from build123d import *

# Parameters (mm, degrees)
SKETCH_1_R      = 1.5
EXTRUDE_1_DEPTH = 14
FILLET_1_R      = 0.5


with BuildPart() as part:
    # 草图1 → 凸台-拉伸1 (new body)
    with BuildSketch(Plane(origin=(0, 0, 0), x_dir=(1, 0, 0), z_dir=(0, 1, 0))):
        Polygon((2.3, -1.327905619), (2.3, 1.327905619), (0, 2.655811238), (-2.3, 1.327905619), (-2.3, -1.327905619), (0, -2.655811238), align=None)
        Circle(SKETCH_1_R, mode=Mode.SUBTRACT)
    extrude(amount=EXTRUDE_1_DEPTH)

    # 圆角1
    fillet_1_edges = [part.edges().sort_by_distance(p)[0] for p in [
        (1.15, 14, -1.991858429),
        (-1.15, 14, -1.991858429),
        (-2.3, 14, 0),
        (-1.15, 14, 1.991858429),
        (1.15, 14, 1.991858429),
        (-1.15, 0, 1.991858429),
        (-2.3, 0, 0),
        (-1.15, 0, -1.991858429),
        (1.15, 0, -1.991858429),
        (2.3, 0, 0),
        (1.15, 0, 1.991858429),
        (2.3, 14, 0),
    ]]
    fillet(fillet_1_edges, radius=FILLET_1_R)


solid = part.part
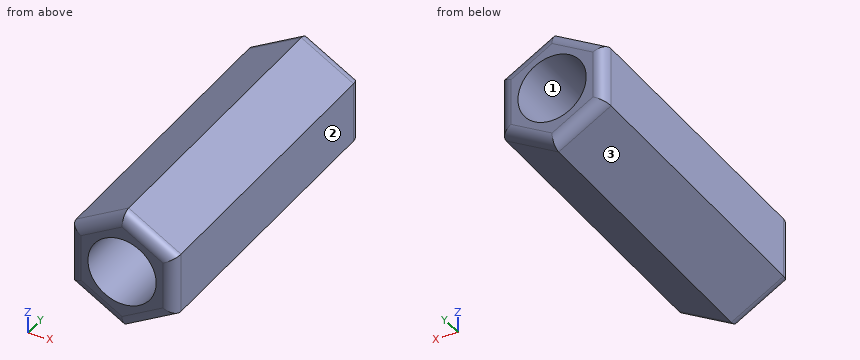
Can you work these out from the model? Positions are in its coordinate system, mm. Face numbers are marked on the shaded views. Coordinates: 2 decimals unless noted, no trailing zeros. Write each loop counter-clockwise with the first axis right and the second up, starting at its lowest first coordinate (ties: lowest second). Pieces come first, ordered by that corner, then holes. Notation, with made-up numbers: (-7, -29) -> (39, -29) arc R32 cw to (39, -2) -> close; hole circle Ø2 at (10.5, 33). An arc over 180 degrees is marked (long way). Write each question's results on one line, items separated by ' | '. Start each with the question number.
Item 1: If we section it at B-B, the plane y = 8: Write out the boundary of the cut face in (x, z).
Item 2: Thinking about a two-plate mould opening in X: for the marked faces 1, 2 and 3, which applies, released by +X, released by -X, zero draft, split by the parting line, or undercut?
Item 3: I'm going to push flat-ended pins straight in: P1, Ø1, axis at y = 11.5, z = 2, coming from the -X side; P2, Ø1, axis at x = 1.5, y = 4, coming from the -Z side; P3, Ø2.5, axis at x = 0, z = 0, coming from the -Y side. Where does each tip first touch, or does it pass through?
Item 4: Please list where these lines run through material, in increasing order: probe 1 along X at (y, z) = (10.5, 0); probe 2 along X at (y, z) = (6.25, -0.7); probe 3 along Z at (x, y) = (-0.05, 4.75).
Item 5: If we section it at A-A, the plane z = 0: Write out the boundary of the cut face in (x, y), and give its area (3 significant figures).
Answer block:
1) outline: (-2.3, -1.33) -> (0, -2.66) -> (2.3, -1.33) -> (2.3, 1.33) -> (0, 2.66) -> (-2.3, 1.33) -> close; hole circle Ø3 at (0, 0)
2) face 1: undercut | face 2: released by +X | face 3: released by -X
3) P1: x = -2 | P2: z = -2.08 | P3: through
4) probe 1: -2.3 to -1.5, 1.5 to 2.3 | probe 2: -2.3 to -1.33, 1.33 to 2.3 | probe 3: -2.63 to -1.5, 1.5 to 2.63
5) outline: (-2.3, 0.5) arc R0.5 ccw to (-1.8, 0) -> (-1.5, 0) -> (-1.5, 14) -> (-1.8, 14) arc R0.5 ccw to (-2.3, 13.5) -> close; (1.5, 0) -> (1.8, 0) arc R0.5 ccw to (2.3, 0.5) -> (2.3, 13.5) arc R0.5 ccw to (1.8, 14) -> (1.5, 14) -> close | area: 22.2 mm²
